Here's how the part is built. I have some questions about the finished solid (model axes, mm). A direction names the side the tool comes from. Round coordinates to 2 decimals unless told otherwise and drop trailing zeros. Loops run counter-clockwise (first coordinate to the right, second up) from the corner with the lowest first, then second, coordinate; pieces in that order, holes last. Notation, with made-up numbers: (69, 81) - (96, 81) arc R9 cw to (96, 91) - close; hole circle Ø1 at (-23, -29). An arc over 180 degrees is marked (long way). Return JSON: item names as keys, results as strings. Group by question number.
```python
from build123d import *

# Parameters (mm, degrees)
F1_DEPTH = 2
F2_DEPTH = 14
F3_W     = 48
F3_H     = 15.884124
F4_DEPTH = 25
F5_R     = 5


with BuildPart() as f1:
    # F0 (on Top) → F1 (new body)
    with BuildSketch(Plane.XY):
        with BuildLine():
            ThreePointArc((37, 65), (34.949747, 69.949747), (30, 72))
            Line((30, 72), (-30, 72))
            ThreePointArc((-30, 72), (-34.949747, 69.949747), (-37, 65))
            Line((-37, 65), (-37, -65))
            ThreePointArc((-37, -65), (-34.949747, -69.949747), (-30, -72))
            Line((-30, -72), (30, -72))
            ThreePointArc((30, -72), (34.949747, -69.949747), (37, -65))
            Line((37, -65), (37, 65))
        make_face()
        with BuildLine():
            Line((-30, 70), (30, 70))
            ThreePointArc((30, 70), (33.535534, 68.535534), (35, 65))
            Line((35, 65), (35, -65))
            ThreePointArc((35, -65), (33.535534, -68.535534), (30, -70))
            Line((30, -70), (-30, -70))
            ThreePointArc((-30, -70), (-33.535534, -68.535534), (-35, -65))
            Line((-35, -65), (-35, 65))
            ThreePointArc((-35, 65), (-33.535534, 68.535534), (-30, 70))
        make_face(mode=Mode.SUBTRACT)
        with BuildLine():
            ThreePointArc((35, 65), (33.535534, 68.535534), (30, 70))
            Line((30, 70), (-30, 70))
            ThreePointArc((-30, 70), (-33.535534, 68.535534), (-35, 65))
            Line((-35, 65), (-35, -65))
            ThreePointArc((-35, -65), (-33.535534, -68.535534), (-30, -70))
            Line((-30, -70), (30, -70))
            ThreePointArc((30, -70), (33.535534, -68.535534), (35, -65))
            Line((35, -65), (35, 65))
        make_face()
    extrude(amount=F1_DEPTH)

    # F0 (on Top) → F2 (join)
    with BuildSketch(Plane.XY):
        with BuildLine():
            ThreePointArc((37, 65), (34.949747, 69.949747), (30, 72))
            Line((30, 72), (-30, 72))
            ThreePointArc((-30, 72), (-34.949747, 69.949747), (-37, 65))
            Line((-37, 65), (-37, -65))
            ThreePointArc((-37, -65), (-34.949747, -69.949747), (-30, -72))
            Line((-30, -72), (30, -72))
            ThreePointArc((30, -72), (34.949747, -69.949747), (37, -65))
            Line((37, -65), (37, 65))
        make_face()
        with BuildLine():
            Line((-30, 70), (30, 70))
            ThreePointArc((30, 70), (33.535534, 68.535534), (35, 65))
            Line((35, 65), (35, -65))
            ThreePointArc((35, -65), (33.535534, -68.535534), (30, -70))
            Line((30, -70), (-30, -70))
            ThreePointArc((-30, -70), (-33.535534, -68.535534), (-35, -65))
            Line((-35, -65), (-35, 65))
            ThreePointArc((-35, 65), (-33.535534, 68.535534), (-30, 70))
        make_face(mode=Mode.SUBTRACT)
    extrude(amount=F2_DEPTH)

    # F3 (on face) → F4 (cut)
    with BuildSketch(Plane.XY.offset(2)):
        with Locations((0, -70)):
            Rectangle(F3_W, F3_H)
    extrude(amount=F4_DEPTH, mode=Mode.SUBTRACT)

    # F5
    f5_edges = [f1.edges().sort_by_distance(p)[0] for p in [
        (-24, -71, 14),
        (24, -71, 14),
    ]]
    fillet(f5_edges, radius=F5_R)


solid = f1.part
```
Q1. If we mould it in two halves opening along X, with no side actions, what happens to faces 4 (the flat face through (-27, -70, 8)), 5 (the cylindrical face through (-35, -69.9, 6.9)), 6 (the cylindrical face through (34.9, -70, 6.9))? For each: +X half, -X half, draft (parallel to the pull), parting line (faces both ways), or undercut.
Q2. Imagine slicing it at B-B, the plane x = -2.5. List the corners of the cut face in (y, z) for me.
Q3. Imagine slicing it at A-A, the plane z = 4.75. List the corners of the cut face in (x, y) for me, and give its area (3 significant figures).
Q4. For faces 1 (the cylindrical face through (33, 69, 8)), 2 (the flat face through (0, 72, 7)), 3 (the cylindrical face through (26, -71, 13)), which set-ups out of +Z, -Z, +X, -X, +Y, -Y let a thin tool reach every point of the face, with its end or its side?
Q5. Imagine slicing it at C-C, the plane y = 13. List the corners of the cut face in (x, z) for me, and give its area (3 significant figures).
Q6. Please list where these lines run through material, in increasing order: line 1 (X direction, y = 15, z = 11.25); line 2 (Y direction, x = 29, z = 11.5); line 3 (Z direction, x = 24.5, y = -36).
Q7. Will these pins go through, and if not, where does the flat tip stop? pin 1 Ø1.5 at (x, z) = (9.5, 7) entering from -Y; pin 2 Ø1.6 at (y, z) = (-71, 6.5) entering from -X; pin 3 Ø0.6 at (y, z) = (-71.5, 5.5) entering from +X.
Q8. Imagine slicing it at D-D, the plane x = 26. List the corners of the cut face in (y, z) for me, and give its area (3 significant figures).
Output values:
{
 "1": {"face 4": "undercut", "face 5": "-X half", "face 6": "+X half"},
 "2": {"outline": "(-72, 0) - (72, 0) - (72, 14) - (70, 14) - (70, 2) - (-72, 2) - close"},
 "3": {"outline": "(-37, -65) arc R7 ccw to (-30, -72) - (-24, -72) - (-24, -70) - (-30, -70) arc R5 cw to (-35, -65) - (-35, 65) arc R5 cw to (-30, 70) - (30, 70) arc R5 cw to (35, 65) - (35, -65) arc R5 cw to (30, -70) - (24, -70) - (24, -72) - (30, -72) arc R7 ccw to (37, -65) - (37, 65) arc R7 ccw to (30, 72) - (-30, 72) arc R7 ccw to (-37, 65) - close", "area": "739 mm^2"},
 "4": {"face 1": "+Z", "face 2": "+Z, -Z, +X, -X, +Y", "face 3": "+Z, -Y"},
 "5": {"outline": "(-37, 0) - (37, 0) - (37, 14) - (35, 14) - (35, 2) - (-35, 2) - (-35, 14) - (-37, 14) - close", "area": "196 mm^2"},
 "6": {"line 1": "x = -37 to -35, 35 to 37", "line 2": "y = -72 to -70, 70 to 72", "line 3": "z = 0 to 2"},
 "7": {"pin 1": "stops at y = 70", "pin 2": "stops at x = -34.69", "pin 3": "stops at x = 33.25"},
 "8": {"outline": "(-72, 0) - (72, 0) - (72, 14) - (70, 14) - (70, 2) - (-70, 2) - (-70, 13) - (-72, 13) - close", "area": "334 mm^2"}
}
